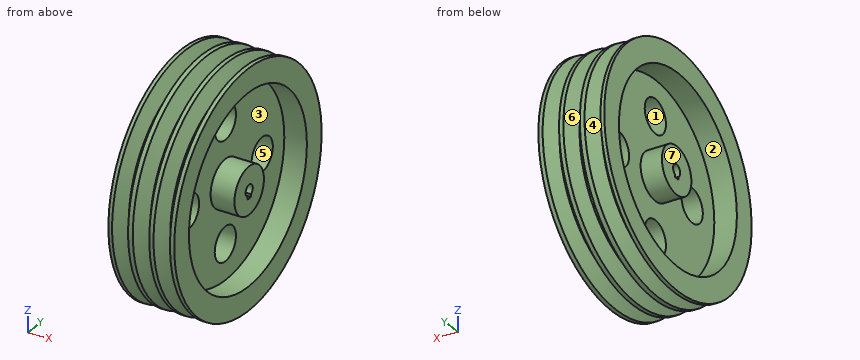
```python
from build123d import *

# Parameters (mm, degrees)
SKETCH1_W              = 22
SKETCH1_H              = 36
SKETCH1_W_2            = 70
SKETCH1_H_2            = 8.416797488
CUT_EXTRUDE2_START     = -70
CUT_EXTRUDE2_OUTLINE_R = 18
CUT_EXTRUDE2_DEPTH     = 70


# Read off the part's stored shape, not the designer's step: Cut-Extrude2
with BuildPart() as part:
    # Sketch1 → Revolve2 (revolve)
    with BuildSketch(Plane(origin=(0, 0, 0), x_dir=(1, 0, 0), z_dir=(0, 1, 0))):
        Polygon((68.651136178, 125), (64.121995326, 125), (57.455679022, 107), (53.089915226, 107), (46.652833964, 125), (42.111811271, 125), (36.118360649, 107), (31.722806927, 107), (24.601983551, 125), (19.601983551, 125), (12.850084898, 107), (8.95007039, 107), (2.597616176, 125), (-1.348863822, 125), (-1.348863822, 100), (22.651136178, 100), (22.651136178, 80.5), (44.651136178, 80.5), (44.651136178, 100), (68.651136178, 100), align=None)
        with Locations((33.651136178, 62.5)):
            Rectangle(SKETCH1_W, SKETCH1_H)
        Polygon((0, 25), (0, 14.5), (70, 14.5), (70, 25), (44.651136178, 25), (44.651136178, 44.5), (22.651136178, 44.5), (22.651136178, 25), align=None)
        with Locations((35, 10.291601256)):
            Rectangle(SKETCH1_W_2, SKETCH1_H_2)
    revolve(axis=Axis((70, 0, 0), (-1, 0, 0)))

    # Cut-Extrude2 outline → Cut-Extrude2 (cut)
    with BuildSketch(Plane(origin=(70, 0, 0), x_dir=(0, 0, -1), z_dir=(1, 0, 0)).offset(CUT_EXTRUDE2_START)):
        with Locations((-62.5, 0)):
            Circle(CUT_EXTRUDE2_OUTLINE_R)
        with Locations((0, -62.5)):
            Circle(CUT_EXTRUDE2_OUTLINE_R)
        with Locations((0, 62.5)):
            Circle(CUT_EXTRUDE2_OUTLINE_R)
        with Locations((62.5, 0)):
            Circle(CUT_EXTRUDE2_OUTLINE_R)
        with BuildLine():
            Line((8.29200839, -3), (8.29200839, 3))
            Line((8.29200839, 3), (5.29200839, 3))
            ThreePointArc((5.29200839, 3), (6.083202512, 0), (5.29200839, -3))
            Line((5.29200839, -3), (8.29200839, -3))
        make_face()
    extrude(amount=CUT_EXTRUDE2_DEPTH, mode=Mode.SUBTRACT)


solid = part.part
```
Part model, mm, in its own coordinate system. Face numbers are marked on the shaded views. A direction names the side the tool comes from. Round coordinates to 2 decimals unless told otherwise and drop trailing zeros.
1. Two-plate mould, pull along X, no slides. Class the marked faces 5, 6 and 7: pulls with the +X half, pulls with the -X half, needs draft (parallel to the pull), parting line crosses it, or undercut.
Solutions:
face 5: needs draft
face 6: undercut
face 7: pulls with the -X half
2. Slice it at A-A (y = -10). Count the separate pieces of the cut face and the enclosed holes in it, and give its area (3 significant figures).
Solutions:
separate pieces: 3
enclosed holes: 0
area: 7,610 mm2
3. Flat gauge pins, fed straight in: pin 1 (3 mm diameter, centred on y = 88, z = 28, fed in from -X); pin 2 (2 mm diameter, centred on x = 45, y = 33.5, fed in from -Z); pin 3 (2.5 mm diameter, centred on x = 24.5, z = -6.5, fed in from -Y). Where does each tip first touch, or does it go through?
Solutions:
pin 1: stops at x = 22.65
pin 2: stops at z = -120.7
pin 3: stops at y = -124.89
4. 3-axis set-ups, long thin cutter, end or side, ignore diameter. For the marked faces 1, 2, 3 and 4: which of +Z, -Z, +X, -X, +Y, -Y reach the whole face in a straight line?
Solutions:
face 1: +X, -X
face 2: -X
face 3: +X
face 4: none
5. Drill centre lines: line 1 along X through (y, z) = (-78, -79); line 2 along X through (y, z) = (33.5, 108.5); line 3 along X through (y, z) = (-71, -60.5). Where is each one in solid material? Low to high.
Solutions:
line 1: x = -1.35 to 7.53, 14.36 to 30.13, 37.46 to 51.65, 58.94 to 68.65
line 2: x = -1.35 to 6.64, 15.31 to 29.13, 38.3 to 50.75, 59.88 to 68.65
line 3: x = 22.65 to 44.65
